Verification items for the finished model (mm, model axes). A direction names the side the tool comes from. Give positions to 0.01 mm unless a question says otherwise; leave off trailing zeros. Order: outer loops, then holes, each group sorted by start corner. A loop starts at its lowest first (then second) coordinate and runs counter-clockwise, first axis right, second up. Notation, with made-up numbers: (68, -12) - (109, -12) arc R27 cw to (109, 20) - close; hole circle Ø3 at (-23, 37). An arc over 180 degrees is marked (long way). Answer as a JSON object with one key per item and string values. Group by question number.
(1) Access from +Z, -Z, +X, -X, +Y, -Y to the whole of each face (thin tool, end or side, straight path). Record for faces 4 (the face through (-57.78, 16.86, 12.52)), 5 (the face through (143.492, 27.788, -63.854)).
(2) Section check B-B (z = 8.5). Record the boundary of the cut face in (x, y), then the cut area to 3 significant figures.
(3) Thickness scan on line 1 (X direction, y = 0, z = 18); line 2 (Y direction, x = 130, z = -59.5); line 3 (X direction, y = -24, z = -13). Record the ranges inside material, lowest first.
(4) Depth check by flat-ended pin: pin 1 Ø6 at (x, z) = (109.5, -57.5) entering from -Y; pin 2 Ø3 at (x, y) = (-31, 6.5) entering from +Z; pin 3 Ø2 at (y, z) = (-6, -11) entering from -X. Enter the tip coordinate at first touch or a pass-through.
(5) Mould release check, pull along Y, two halves, no side actions. Record for faces 1 (the face through (68.836, 27.054, -54.575)), 2 (the face through (-60.724, 19.123, 12.522)), 3 (the face through (-36, -28, 25.4)): +Y half, -Y half, draft (parallel to the pull), parting line (faces both ways), or undercut.
(6) Section check C-C (y = -19). Record the boundary of the cut face in (x, z).
(7) Section check A-A (y = 24). Record the boundary of the cut face in (x, z), then the cut area to 3 significant figures.
```python
from build123d import *

# Parameters (mm, degrees)
F1_R   = 31.4265848645
F1_R_2 = 27.7125712081


# Not quite as in the source:
# - the program builds the solid bodies; features that only make, move or delete a surface that nothing else refers to are left out


with BuildPart() as f2:
    # F2: sweep along a path in F0
    with BuildLine(Plane.XZ) as f2_path:
        Line((-35.56, 25.4), (-35.56, 0))
        ThreePointArc((-35.56, 0), (-27.2405403973, -22.8575274005), (-6.1749291978, -35.0197636971))
        Line((-6.1749291978, -35.0197636971), (143.9097723612, -61.4837459736))
    # F1 (on Top) → F2 (sweep)
    with BuildSketch(Plane.XY):
        with Locations((-35.7853956521, 0)):
            Circle(F1_R)
        with Locations((-35.7853956521, 0)):
            Circle(F1_R_2, mode=Mode.SUBTRACT)
    sweep(path=f2_path.line)


solid = f2.part
```
Solutions:
{
 "1": {"face 4": "+Z", "face 5": "-Z, +X, +Y, -Y"},
 "2": {"outline": "circle Ø62.85 at (-35.79, 0); hole circle Ø55.43 at (-35.79, 0)", "area": "690 mm2"},
 "3": {"line 1": "x = -67.21 to -63.5, -8.07 to -4.36", "line 2": "y = -31.43 to -27.71, 27.71 to 31.43", "line 3": "x = -54.55 to -47.91, -17.66 to -8.43"},
 "4": {"pin 1": "stops at y = -31.43", "pin 2": "stops at z = -53.54", "pin 3": "stops at x = -65.97"},
 "5": {"face 1": "undercut", "face 2": "parting line", "face 3": "draft"},
 "6": {"outline": "(-60.82, 0) arc R60.82 ccw to (-10.56, -59.89) - (139.52, -86.36) - (140.37, -81.57) - (-9.72, -55.11) arc R55.96 cw to (-55.96, 0) - (-55.96, 25.4) - (-60.82, 25.4) - close; (-15.61, 0) arc R15.61 ccw to (-2.71, -15.37) - (147.37, -41.84) - (148.22, -37.05) - (-1.87, -10.59) arc R10.75 cw to (-10.75, 0) - (-10.75, 25.4) - (-15.61, 25.4) - close"},
 "7": {"outline": "(-56.07, 0) arc R56.07 ccw to (-9.74, -55.22) - (140.35, -81.69) - (141.46, -75.35) - (-8.62, -48.89) arc R49.64 cw to (-49.64, 0) - (-49.64, 25.4) - (-56.07, 25.4) - close; (-21.93, 0) arc R21.93 ccw to (-3.81, -21.6) - (146.28, -48.06) - (147.39, -41.73) - (-2.69, -15.26) arc R15.5 cw to (-15.5, 0) - (-15.5, 25.4) - (-21.93, 25.4) - close", "area": "2,930 mm2"}
}
